Here's how the part is built. I have some questions about the finished solid (model axes, mm). Coordinates: 2 decimals unless noted, no trailing zeros. Use a Markdown table: item, result.
```python
from build123d import *

# Parameters (mm, degrees)
SKETCH1_R      = 3.4036
EXTRUDE1_DEPTH = 300


with BuildPart() as part:
    # Sketch1 → Extrude1 (new body)
    with BuildSketch(Plane.XY):
        with BuildLine():
            Line((-20, 6.825), (-20, -6.825))
            ThreePointArc((-20, -6.825), (-19.07006403, -9.07006403), (-16.825, -10))
            Line((-16.825, -10), (16.825, -10))
            ThreePointArc((16.825, -10), (19.07006403, -9.07006403), (20, -6.825))
            Line((20, -6.825), (20, 6.825))
            ThreePointArc((20, 6.825), (19.07006403, 9.07006403), (16.825, 10))
            Line((16.825, 10), (13.01772333, 10))
            Line((13.01772333, 10), (5.624351215, 10))
            ThreePointArc((5.624351215, 10), (4.518187863, 9.541812137), (4.06, 8.435648785))
            Line((4.06, 8.435648785), (4.06, 7.5148))
            ThreePointArc((4.06, 7.5148), (4.521248241, 6.401248241), (5.6348, 5.94))
            Line((5.6348, 5.94), (6.771827505, 5.94))
            Line((6.771827505, 5.94), (6.771827505, 6.708913257))
            Line((6.771827505, 6.708913257), (9.01577365, 6.708913257))
            ThreePointArc((9.01577365, 6.708913257), (9.929335196, 6.321129388), (10.285, 5.394590897))
            Line((10.285, 5.394590897), (10.285, 3.096216247))
            ThreePointArc((10.285, 3.096216247), (10.241244142, 2.808525014), (10.106931233, 2.550376096))
            Line((10.106931233, 2.550376096), (6.737817619, -0.818737518))
            ThreePointArc((6.737817619, -0.818737518), (5.207385794, -1.896930484), (3.37920183, -2.3))
            Line((3.37920183, -2.3), (-3.37920183, -2.3))
            ThreePointArc((-3.37920183, -2.3), (-5.207385794, -1.896930484), (-6.737817619, -0.818737518))
            Line((-6.737817619, -0.818737518), (-10.024617928, 2.468062791))
            ThreePointArc((-10.024617928, 2.468062791), (-10.217328904, 2.756475149), (-10.285, 3.09668072))
            Line((-10.285, 3.09668072), (-10.285, 5.394590897))
            ThreePointArc((-10.285, 5.394590897), (-9.929335196, 6.321129388), (-9.01577365, 6.708913257))
            Line((-9.01577365, 6.708913257), (-6.771827505, 6.708913257))
            Line((-6.771827505, 6.708913257), (-6.771827505, 5.94))
            Line((-6.771827505, 5.94), (-5.6348, 5.94))
            ThreePointArc((-5.6348, 5.94), (-4.521248241, 6.401248241), (-4.06, 7.5148))
            Line((-4.06, 7.5148), (-4.06, 8.435648785))
            ThreePointArc((-4.06, 8.435648785), (-4.518187863, 9.541812137), (-5.624351215, 10))
            Line((-5.624351215, 10), (-13.017278808, 10))
            Line((-13.017278808, 10), (-16.825, 10))
            ThreePointArc((-16.825, 10), (-19.07006403, 9.07006403), (-20, 6.825))
        make_face()
        with Locations((-14, -4)):
            Circle(SKETCH1_R, mode=Mode.SUBTRACT)
        with Locations((14, -4)):
            Circle(SKETCH1_R, mode=Mode.SUBTRACT)
        with BuildLine():
            Line((-13.212346722, 1.939194793), (-17.688897149, 1.939194793))
            ThreePointArc((-17.688897149, 1.939194793), (-18.133514414, 2.127552649), (-18.31710748, 2.574158493))
            Line((-18.31710748, 2.574158493), (-18.31710748, 5.56561917))
            ThreePointArc((-18.31710748, 5.56561917), (-17.477686114, 7.532412526), (-15.493392654, 8.329584904))
            Line((-15.493392654, 8.329584904), (-12.501931977, 8.329584904))
            ThreePointArc((-12.501931977, 8.329584904), (-12.097931082, 8.115619133), (-11.942346722, 7.68574522))
            Line((-11.942346722, 7.68574522), (-11.942346722, 3.209194793))
            ThreePointArc((-11.942346722, 3.209194793), (-12.31432111, 2.31116918), (-13.212346722, 1.939194793))
        make_face(mode=Mode.SUBTRACT)
        with BuildLine():
            Line((18.32404339, 5.503747464), (18.32404339, 2.512286787))
            ThreePointArc((18.32404339, 2.512286787), (18.11465108, 2.106331374), (17.686957075, 1.945948162))
            Line((17.686957075, 1.945948162), (13.210406647, 1.945948162))
            ThreePointArc((13.210406647, 1.945948162), (12.312381035, 2.31792255), (11.940406647, 3.215948162))
            Line((11.940406647, 3.215948162), (11.940406647, 7.692498589))
            ThreePointArc((11.940406647, 7.692498589), (12.123999713, 8.139104433), (12.568616978, 8.327462289))
            Line((12.568616978, 8.327462289), (15.560077655, 8.327462289))
            ThreePointArc((15.560077655, 8.327462289), (17.526871011, 7.488040923), (18.32404339, 5.503747464))
        make_face(mode=Mode.SUBTRACT)
    extrude(amount=-EXTRUDE1_DEPTH)


solid = part.part
```
1. We'd pull the mould along X, two halves only. Please class faces 1 (the face through (20, 0, -148)), 2 (the face through (-20, 0, -148)), 3 (the face through (0, -2.3, -148)), 4 (the face through (0, -10, -148)): +X half, -X half, draft (parallel to the pull), parting line (faces both ways), or undercut.
Answers follow:
| item | result |
|---|---|
| face 1 | +X half |
| face 2 | -X half |
| face 3 | undercut |
| face 4 | draft |
2. Will these pins go through, and if not, where does the flat tip stop? pin 1 Ø7.5 at (x, z) = (-0.5, -131.5) entering from +Y; pin 2 Ø0.5 at (y, z) = (8, -88) entering from +X; pin 3 Ø5 at (x, y) = (-2, 1.5) entering from +Z; pin 4 Ø1 at (y, z) = (8, -151.5) entering from -X.
Answers follow:
| item | result |
|---|---|
| pin 1 | stops at y = 9.18 |
| pin 2 | stops at x = 19.86 |
| pin 3 | passes through |
| pin 4 | stops at x = -19.93 |
3. Suppose I cut it at A-A on z = -87.5. State how many separate pieces and enclosed holes the cut face has, and give its area (3 significant figures).
Answers follow:
| item | result |
|---|---|
| separate pieces | 1 |
| enclosed holes | 4 |
| area | 458 mm2 |
4. I need wall thicknesses on probe 1 along Y at (x, z) = (14, -79); probe 2 along X at (y, z) = (4.25, -164.5) (3 decimals); probe 3 along Y at (x, z) = (-16, -147.5). Which ranges of each line are inside material? Lowest first, please.
Answers follow:
| item | result |
|---|---|
| probe 1 | y = -10 to -7.4, -0.6 to 1.95, 8.33 to 10 |
| probe 2 | x = -20 to -18.317, -11.942 to -10.285, 10.285 to 11.94, 18.324 to 20 |
| probe 3 | y = -10 to -6.75, -1.25 to 1.94, 8.29 to 10 |
